Verification items for the finished model (mm, model axes). Face numbers are marked on the shaded views. A direction names the side the tool comes from. Round coordinates to 2 decimals unless told otherwise and drop trailing zeros. Loops run counter-clockwise (first coordinate to the right, second up) from the corner with the lowest first, then second, coordinate; pieces in that order, holes last. Notation, with made-up numbers: M 58,31 L 66,31 A22 cw 66,51 Z; hole C 22,-26 d2. An arc over 180 degrees is marked long. Answer as CSV lines item,"result".
```python
from build123d import *

# Parameters (mm, degrees)
SKETCH1_W           = 25
SKETCH1_H           = 25
BOSS_EXTRUDE1_DEPTH = 5
SKETCH2_W           = 25
SKETCH2_H           = 8
BOSS_EXTRUDE2_DEPTH = 50
SKETCH3_W           = 25
SKETCH3_H           = 20
BOSS_EXTRUDE3_DEPTH = 30


with BuildPart() as part:
    # Sketch1 → Boss-Extrude1 (new body)
    with BuildSketch(Plane(origin=(0, 0, 0), x_dir=(1, 0, 0), z_dir=(0, 1, 0))):
        Rectangle(SKETCH1_W, SKETCH1_H)
    extrude(amount=BOSS_EXTRUDE1_DEPTH)

    # Sketch2 → Boss-Extrude2 (add)
    with BuildSketch(Plane(origin=(0, 5, 0), x_dir=(1, 0, 0), z_dir=(0, 1, 0))):
        with Locations((0, -8.5)):
            Rectangle(SKETCH2_W, SKETCH2_H)
    extrude(amount=BOSS_EXTRUDE2_DEPTH)

    # Sketch3 → Boss-Extrude3 (add)
    with BuildSketch(Plane.XY.offset(12.5)):
        with Locations((0, 45)):
            Rectangle(SKETCH3_W, SKETCH3_H)
    extrude(amount=BOSS_EXTRUDE3_DEPTH)


solid = part.part
```
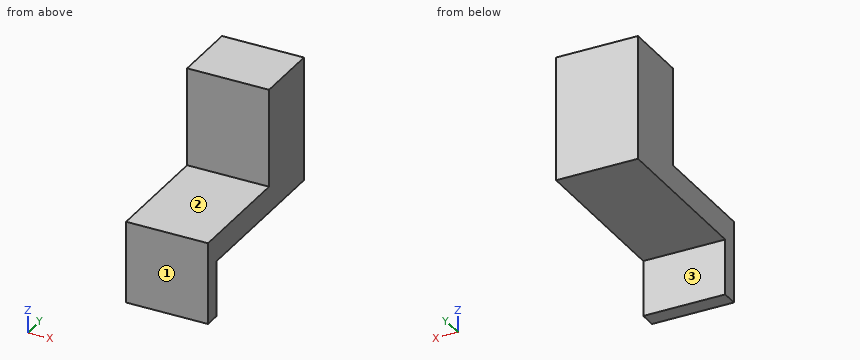
1) Set-up check for the marked faces 1, 2 and 3: record each of +Z, -Z, +X, -X, +Y, -Y from which the full face is reachable in a straight line by a thin tool's end or side.
Here are the results:
face 1,"+Z, -Z, +X, -X, -Y"
face 2,"+Z, +X, -X, -Y"
face 3,"-Z, +X, -X, +Y"
2) Go/stop test with flat-tipped pins: pin 1 (3 mm diameter, centred on x = -4, y = 25, fed in from +Z); pin 2 (1 mm diameter, centred on x = 0, z = 13.5, fed in from -Y); pin 3 (4 mm diameter, centred on x = 9.5, z = 0, fed in from -Y); pin 4 (5 mm diameter, centred on x = 0, z = -0.5, fed in from +Y). Record where each tip stops, or that it passes through.
Here are the results:
pin 1,"stops at z = 12.5"
pin 2,"stops at y = 35"
pin 3,"stops at y = 0"
pin 4,"stops at y = 5"
3) Section check C-C (y = 45.5). Record the cut outline in (x, z), plus the area to 3 significant figures.
Here are the results:
outline,"M -12.5,4.5 L 12.5,4.5 L 12.5,42.5 L -12.5,42.5 Z"
area,"950 mm^2"
4) Section check A-A (x = -2). Record the cut outline in (y, z), plus the area to 4 significant figures.
Here are the results:
outline,"M 0,-12.5 L 5,-12.5 L 5,4.5 L 55,4.5 L 55,42.5 L 35,42.5 L 35,12.5 L 0,12.5 Z"
area,"1,125 mm^2"
5) Section check B-B (z = 33). Record the cut outline in (x, y), plus the area to 3 significant figures.
Here are the results:
outline,"M -12.5,35 L 12.5,35 L 12.5,55 L -12.5,55 Z"
area,"500 mm^2"
6) Material ranges on probe 1 along Y at (x, z) = (8.25, 28.5); probe 2 along Z at (x, y) = (2.5, 30); probe 3 along Y at (x, z) = (4.25, -5.5), recorded low to high.
Here are the results:
probe 1,"y = 35 to 55"
probe 2,"z = 4.5 to 12.5"
probe 3,"y = 0 to 5"
